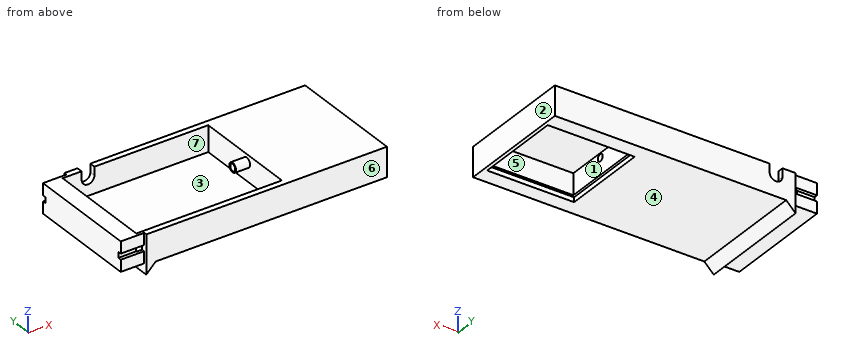
```python
from build123d import *

# Parameters (mm, degrees)
SKETCH1_W           = 170
SKETCH1_H           = 100
BOSS_EXTRUDE1_DEPTH = 15
SKETCH3_W           = 70
SKETCH3_H           = 90
CUT_EXTRUDE2_DEPTH  = 12
SKETCH8_W           = 15
SKETCH8_H           = 15
CUT_EXTRUDE9_DEPTH  = 2.5
SKETCH9_W           = 15
SKETCH9_H           = 15
CUT_EXTRUDE10_DEPTH = 2.5
SKETCH10_W          = 12
SKETCH10_H          = 90
CUT_EXTRUDE11_DEPTH = 58
SKETCH11_W          = 128
SKETCH11_H          = 90
BOSS_EXTRUDE2_DEPTH = 10
SKETCH12_W          = 22
SKETCH12_H          = 90
BOSS_EXTRUDE4_DEPTH = 4
BOSS_EXTRUDE6_DEPTH = 100
SKETCH15_W          = 5
SKETCH15_H          = 3
CUT_EXTRUDE14_DEPTH = 15
SKETCH16_W          = 25
SKETCH16_H          = 100
BOSS_EXTRUDE7_DEPTH = 50
SKETCH17_W          = 70
SKETCH17_H          = 70
CUT_EXTRUDE15_DEPTH = 22
SKETCH18_W          = 74
SKETCH18_H          = 74
SKETCH18_W_2        = 70
SKETCH18_H_2        = 70
CUT_EXTRUDE16_DEPTH = 4
BOSS_EXTRUDE8_DEPTH = 5
SKETCH20_R          = 4
SKETCH20_R_2        = 3
BOSS_EXTRUDE9_DEPTH = 23
SKETCH20_2_R        = 3
CUT_EXTRUDE17_DEPTH = 23
CUT_EXTRUDE18_DEPTH = 23


with BuildPart() as part:
    # Sketch1 → Boss-Extrude1 (new body)
    with BuildSketch(Plane.XY):
        with Locations((-16.108033241, 2.077562327)):
            Rectangle(SKETCH1_W, SKETCH1_H)
    extrude(amount=BOSS_EXTRUDE1_DEPTH)

    # Sketch3 → Cut-Extrude2 (cut)
    with BuildSketch(Plane.XY.offset(15)):
        with Locations((-56.108033241, 2.077562327)):
            Rectangle(SKETCH3_W, SKETCH3_H)
    extrude(amount=-CUT_EXTRUDE2_DEPTH, mode=Mode.SUBTRACT)

    # Sketch8 → Cut-Extrude9 (cut)
    with BuildSketch(Plane(origin=(0, 52.077562327, 0), x_dir=(1, 0, 0), z_dir=(0, 1, 0))):
        with Locations((-93.608033241, -7.5)):
            Rectangle(SKETCH8_W, SKETCH8_H)
    extrude(amount=-CUT_EXTRUDE9_DEPTH, mode=Mode.SUBTRACT)

    # Sketch9 → Cut-Extrude10 (cut)
    with BuildSketch(Plane.XZ.offset(47.922437673)):
        with Locations((-93.608033241, 7.5)):
            Rectangle(SKETCH9_W, SKETCH9_H)
    extrude(amount=-CUT_EXTRUDE10_DEPTH, mode=Mode.SUBTRACT)

    # Sketch10 → Cut-Extrude11 (cut)
    with BuildSketch(Plane.ZY.offset(21.108033241)):
        with Locations((9, 2.077562327)):
            Rectangle(SKETCH10_W, SKETCH10_H)
    extrude(amount=-CUT_EXTRUDE11_DEPTH, mode=Mode.SUBTRACT)

    # Sketch11 → Boss-Extrude2 (add)
    with BuildSketch(Plane.XY.offset(15)):
        Polygon((-86.108033241, -45.422437673), (-86.108033241, -47.922437673), (68.891966759, -47.922437673), (68.891966759, 52.077562327), (-86.108033241, 52.077562327), (-86.108033241, 49.577562327), (-101.108033241, 49.577562327), (-101.108033241, -45.422437673), align=None)
        with Locations((-27.108033241, 2.077562327)):
            Rectangle(SKETCH11_W, SKETCH11_H, mode=Mode.SUBTRACT)
    extrude(amount=BOSS_EXTRUDE2_DEPTH)

    # Sketch12 → Boss-Extrude4 (add)
    with BuildSketch(Plane.ZY.offset(-36.891966759)):
        with Locations((14, 2.077562327)):
            Rectangle(SKETCH12_W, SKETCH12_H)
    extrude(amount=BOSS_EXTRUDE4_DEPTH)

    # Sketch14 → Boss-Extrude6 (add)
    with BuildSketch(Plane(origin=(0, 52.077562327, 0), x_dir=(1, 0, 0), z_dir=(0, 1, 0))):
        Polygon((-86.108033241, 0), (-78.108033241, 0), (-86.108033241, 8), align=None)
    extrude(amount=-BOSS_EXTRUDE6_DEPTH)

    # Sketch15 → Cut-Extrude14 (cut)
    with BuildSketch(Plane.ZY.offset(101.108033241)):
        with Locations((12.5, 48.077562327)):
            Rectangle(SKETCH15_W, SKETCH15_H)
        with Locations((12.5, -43.922437673)):
            Rectangle(SKETCH15_W, SKETCH15_H)
    extrude(amount=-CUT_EXTRUDE14_DEPTH, mode=Mode.SUBTRACT)

    # Sketch16 → Boss-Extrude7 (add)
    with BuildSketch(Plane(origin=(68.891966759, 0, 0), x_dir=(0, 0, -1), z_dir=(1, 0, 0))):
        with Locations((-12.5, 2.077562327)):
            Rectangle(SKETCH16_W, SKETCH16_H)
    extrude(amount=BOSS_EXTRUDE7_DEPTH)

    # Sketch17 → Cut-Extrude15 (cut)
    with BuildSketch(Plane(origin=(0, 0, 0), x_dir=(-1, 0, 0), z_dir=(0, 0, -1))):
        with Locations((-78.891966759, 2.077562327)):
            Rectangle(SKETCH17_W, SKETCH17_H)
    extrude(amount=-CUT_EXTRUDE15_DEPTH, mode=Mode.SUBTRACT)

    # Sketch18 → Cut-Extrude16 (cut)
    with BuildSketch(Plane(origin=(0, 0, 0), x_dir=(-1, 0, 0), z_dir=(0, 0, -1))):
        with Locations((-78.891966759, 2.077562327)):
            Rectangle(SKETCH18_W, SKETCH18_H)
        with Locations((-78.891966759, 2.077562327)):
            Rectangle(SKETCH18_W_2, SKETCH18_H_2, mode=Mode.SUBTRACT)
    extrude(amount=-CUT_EXTRUDE16_DEPTH, mode=Mode.SUBTRACT)

    # Sketch19 → Boss-Extrude8 (add)
    with BuildSketch(Plane.ZY.offset(101.108033241)):
        Polygon((10, 46.577562327), (10, 49.577562327), (0, 49.577562327), (0, -45.422437673), (10, -45.422437673), (10, -42.422437673), (15, -42.422437673), (15, -45.422437673), (25, -45.422437673), (25, 49.577562327), (15, 49.577562327), (15, 46.577562327), align=None)
    extrude(amount=BOSS_EXTRUDE8_DEPTH)

    # Sketch20 → Boss-Extrude9 (add)
    with BuildSketch(Plane(origin=(43.891966759, 0, 0), x_dir=(0, 0, -1), z_dir=(1, 0, 0))):
        with Locations((-18.181884359, 0)):
            Circle(SKETCH20_R)
        with Locations((-18.181884359, 0)):
            Circle(SKETCH20_R_2, mode=Mode.SUBTRACT)
    extrude(amount=-BOSS_EXTRUDE9_DEPTH)

    # Sketch20<2> → Cut-Extrude17 (cut)
    with BuildSketch(Plane(origin=(43.891966759, 0, 0), x_dir=(0, 0, -1), z_dir=(1, 0, 0))):
        with Locations((-18.181884359, 0)):
            Circle(SKETCH20_2_R)
    extrude(amount=-CUT_EXTRUDE17_DEPTH, mode=Mode.SUBTRACT)

    # Sketch21 → Cut-Extrude18 (cut)
    with BuildSketch(Plane(origin=(0, 52.077562327, 0), x_dir=(1, 0, 0), z_dir=(0, 1, 0))):
        with BuildLine():
            Line((-74.929235075, -25), (-74.929235075, -17.797726587))
            ThreePointArc((-74.929235075, -17.797726587), (-69.494183986, -12.362675498), (-64.059132898, -17.797726587))
            Line((-64.059132898, -17.797726587), (-64.059132898, -25))
            ThreePointArc((-64.059132898, -25), (-69.494183986, -30.435051089), (-74.929235075, -25))
        make_face()
    extrude(amount=-CUT_EXTRUDE18_DEPTH, mode=Mode.SUBTRACT)


solid = part.part
```
Here's how the part is built. I have some questions about the finished solid (model axes, mm). Face numbers are marked on the shaded views. A direction names the side the tool comes from. Coordinates: 2 decimals unless noted, no trailing zeros. Order: outer loops, then holes, each group sorted by start corner. A loop starts at its lowest first (then second) coordinate and runs counter-clockwise, first axis right, second up.
1) Will these pins go through, and if not, where does the flat tip stop? pin 1 (1.5 mm diameter, centred on x = -95.5, z = 11.5, fed in from +Y); pin 2 (11 mm diameter, centred on x = -99.5, z = 19, fed in from -Y); pin 3 (16 mm diameter, centred on x = -98.5, y = 17, fed in from -Z).
2) I need wall thicknesses on line 1 (X direction, y = -0.5, z = 6.5); line 2 (Y direction, x = 47, z = 0.5); line 3 (Y direction, x = -24.5, z = 14.5). Which ranges of each line are inside material? Lowest first, please.
3) Imagine slicing it at C-C on y = -23.5. List the corners of the cut face in (x, z) for me, and give its area (3 significant figures).
4) We'd pull the mould along X, two halves only. Please class the marked faces 1, 2, 3 and 4: +X half, -X half, draft (parallel to the pull), parting line (faces both ways), or undercut.
5) Imagine slicing it at D-D on x = 104.5. List the corners of the cut face in (y, z) for me.
6) Imagine slicing it at A-A on x = 7. List the corners of the cut face in (y, z) for me, and give its area (3 significant figures).
7) Imagine slicing it at B-B on y = 0. List the corners of the cut face in (x, z) for me.
8) Which directions (+Z, -Z, +X, -X, +Y, -Y) give clear straight access to the entire face, cutting with the end or side of a thin tool? Please do the marked faces 5, 6 and 7.
Response values:
1. pin 1: stops at y = 46.58
1. pin 2: stops at y = -45.42
1. pin 3: stops at z = 0
2. line 1: x = -106.11 to -91.11, 32.89 to 43.89, 113.89 to 118.89
2. line 2: y = -47.92 to -34.92, 39.08 to 52.08
2. line 3: y = -47.92 to -42.92, 47.08 to 52.08
3. outline: (-106.11, 0) - (-86.11, 0) - (-86.11, -8) - (-78.11, 0) - (41.89, 0) - (41.89, 4) - (43.89, 4) - (43.89, 22) - (113.89, 22) - (113.89, 4) - (115.89, 4) - (115.89, 0) - (118.89, 0) - (118.89, 25) - (32.89, 25) - (32.89, 3) - (-91.11, 3) - (-91.11, 25) - (-106.11, 25) - close
3. area: 1,370 mm2
4. face 1: undercut
4. face 2: +X half
4. face 3: undercut
4. face 4: draft
5. outline: (-47.92, 0) - (-34.92, 0) - (-34.92, 4) - (-32.92, 4) - (-32.92, 22) - (37.08, 22) - (37.08, 4) - (39.08, 4) - (39.08, 0) - (52.08, 0) - (52.08, 25) - (-47.92, 25) - close
6. outline: (-47.92, 0) - (52.08, 0) - (52.08, 25) - (47.08, 25) - (47.08, 3) - (-42.92, 3) - (-42.92, 25) - (-47.92, 25) - close
6. area: 520 mm2
7. outline: (-106.11, 0) - (-86.11, 0) - (-86.11, -8) - (-78.11, 0) - (41.89, 0) - (41.89, 4) - (43.89, 4) - (43.89, 15.18) - (20.89, 15.18) - (20.89, 14.18) - (32.89, 14.18) - (32.89, 3) - (-91.11, 3) - (-91.11, 25) - (-106.11, 25) - close; (20.89, 21.18) - (43.89, 21.18) - (43.89, 22) - (113.89, 22) - (113.89, 4) - (115.89, 4) - (115.89, 0) - (118.89, 0) - (118.89, 25) - (32.89, 25) - (32.89, 22.18) - (20.89, 22.18) - close
8. face 5: -Z
8. face 6: +Z, -Z, +X, -X, -Y
8. face 7: +Z
